The listing builds one solid part. Answer for the finished solid, in the listing's coordinates (mm). Face numbers are marked on the shaded views. A direction names the side the tool comes from. Give positions to 0.01 mm unless a question says otherwise; leave off trailing zeros. Loops run counter-clockwise (first coordinate to the right, second up) from the corner with the lowest first, then second, coordinate; pieces in that order, holes last. Notation, with made-up numbers: M -19,54 L -10,54 A16 cw -10,80 Z; hole C 61.5,75 d1. An arc over 180 degrees is marked long. Return JSON: item names as keys, results as strings.
from build123d import *

# Parameters (mm, degrees)
SKETCH1_R           = 1
BOSS_EXTRUDE1_DEPTH = 6
SKETCH2_R           = 0.25
BOSS_EXTRUDE2_DEPTH = 4


with BuildPart() as part:
    # Sketch1 → Boss-Extrude1 (new body, symmetric)
    with BuildSketch(Plane.XY):
        Circle(SKETCH1_R)
    extrude(amount=BOSS_EXTRUDE1_DEPTH, both=True)

    # Sketch2 → Boss-Extrude2 (add)
    with BuildSketch(Plane(origin=(0, 0, 0), x_dir=(1, 0, 0), z_dir=(0, 1, 0))):
        with Locations((0, -6)):
            Circle(SKETCH2_R)
        with Locations((0, 6)):
            Circle(SKETCH2_R)
    extrude(amount=BOSS_EXTRUDE2_DEPTH)


solid = part.part
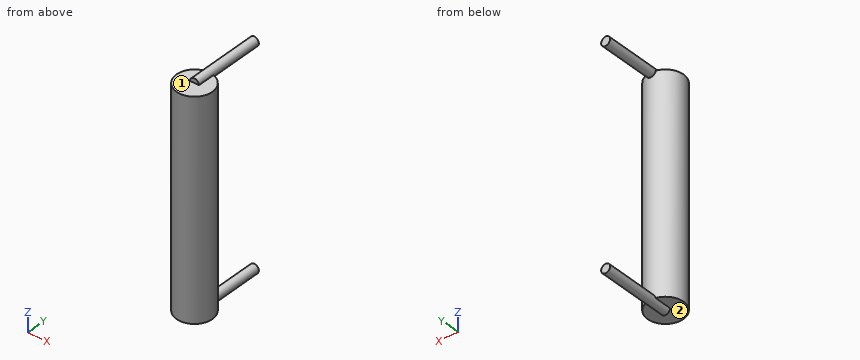
(1) The part is cut by section B-B (y = 2.95). Determine the outline of the cut face in (x, z), and give its area (3 significant figures).
Values follow:
{"outline": "C 0,-6 d0.5; C 0,6 d0.5", "area": "0.393 mm²"}
(2) The part is cut by section A-A (x = 0). Determine the outline of the cut face in (y, z).
Values follow:
{"outline": "M -1,-6 L 0,-6 L 0,-6.25 L 4,-6.25 L 4,-5.75 L 1,-5.75 L 1,5.75 L 4,5.75 L 4,6.25 L 0,6.25 L 0,6 L -1,6 Z"}
(3) The part is cut by section D-D (y = 0.85). Determine the outline of the cut face in (x, z).
Values follow:
{"outline": "M -0.53,-6 L -0.25,-6 A0.25 ccw 0.25,-6 L 0.53,-6 L 0.53,6 L 0.25,6 A0.25 ccw -0.25,6 L -0.53,6 Z"}
(4) The part is cut by section C-C (z = 3.75). Determine the outline of the cut face in (x, y).
Values follow:
{"outline": "C 0,0 d2"}
(5) A tool of negligible diameter and unlimited length cuts with its end or side. For the marked faces 1 and 2, from which of +Z, -Z, +X, -X, +Y, -Y can it reach the whole face along a straight path? Write none if from no direction.
Values follow:
{"face 1": "+Z, -Y", "face 2": "-Z, -Y"}
(6) Straight lines are drawn through the part: line 1 along Z through (x, y) = (0, 3.55); line 2 along Z through (x, y) = (0.5, -0.4); line 3 along X through (y, z) = (0.2, 0.25). For each, find the intervals that lie inside material, in ascending order.
Values follow:
{"line 1": "-6.25 to -5.75, 5.75 to 6.25", "line 2": "-6 to 6", "line 3": "-0.98 to 0.98"}
